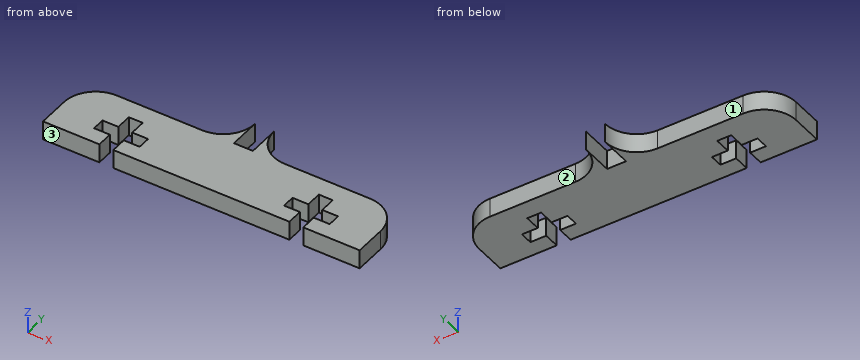
```python
from build123d import *

# Parameters (mm, degrees)
BOSS_EXTRUDE1_DEPTH = 3
FILLET1_R           = 5


with BuildPart() as part:
    # Sketch1 → Boss-Extrude1 (new body)
    with BuildSketch(Plane.XY):
        with BuildLine():
            Line((-25, -5), (-16.1, -5))
            Line((-16.1, -5), (-16.1, -2.5))
            Line((-16.1, -2.5), (-18.6, -2.5))
            Line((-18.6, -2.5), (-18.6, -0.5))
            Line((-18.6, -0.5), (-16.1, -0.5))
            Line((-16.1, -0.5), (-16.1, 2))
            Line((-16.1, 2), (-13.9, 2))
            Line((-13.9, 2), (-13.9, -0.5))
            Line((-13.9, -0.5), (-11.4, -0.5))
            Line((-11.4, -0.5), (-11.4, -2.5))
            Line((-11.4, -2.5), (-13.9, -2.5))
            Line((-13.9, -2.5), (-13.9, -5))
            Line((-13.9, -5), (13.9, -5))
            Line((13.9, -5), (13.9, -2.5))
            Line((13.9, -2.5), (11.4, -2.5))
            Line((11.4, -2.5), (11.4, -0.5))
            Line((11.4, -0.5), (13.9, -0.5))
            Line((13.9, -0.5), (13.9, 2))
            Line((13.9, 2), (16.1, 2))
            Line((16.1, 2), (16.1, -0.5))
            Line((16.1, -0.5), (18.6, -0.5))
            Line((18.6, -0.5), (18.6, -2.5))
            Line((18.6, -2.5), (16.1, -2.5))
            Line((16.1, -2.5), (16.1, -5))
            Line((16.1, -5), (25, -5))
            Line((25, -5), (25, 5))
            Line((25, 5), (6.5, 5))
            ThreePointArc((6.5, 5), (2.964466094, 6.464466094), (1.5, 10))
            Line((1.5, 10), (1.5, 5))
            Line((1.5, 5), (-1.5, 5))
            Line((-1.5, 5), (-1.5, 10))
            ThreePointArc((-1.5, 10), (-2.964466094, 6.464466094), (-6.5, 5))
            Line((-6.5, 5), (-25, 5))
            Line((-25, 5), (-25, -5))
        make_face()
    extrude(amount=BOSS_EXTRUDE1_DEPTH)

    # Fillet1
    fillet1_edges = [part.edges().sort_by_distance(p)[0] for p in [
        (25, 5, 1.5),
        (-25, 5, 1.5),
    ]]
    fillet(fillet1_edges, radius=FILLET1_R)


solid = part.part
```
For this review, take the finished solid that the model builds, in its own axes (mm). Face numbers are marked on the shaded views. A direction names the side the tool comes from. Give positions to 0.01 mm unless a question says otherwise; leave off trailing zeros. Write each loop counter-clockwise with the first axis right and the second up, starting at its lowest first coordinate (ties: lowest second). Pieces come first, ordered by that corner, then holes. Notation, with made-up numbers: M 59.25,17 L 82.25,17 A24 ccw 82.25,40 Z; hole C -4.5,-38 d5. An arc over 180 degrees is marked long. Answer as CSV lines item,"result".
1. Consider section D-D, the plane y = -4. Write out the cut boundary in (x, z), then the cut area to 3 significant figures.
Findings:
outline,"M -25,0 L -16.1,0 L -16.1,3 L -25,3 Z; M -13.9,0 L 13.9,0 L 13.9,3 L -13.9,3 Z; M 16.1,0 L 25,0 L 25,3 L 16.1,3 Z"
area,"137 mm2"
2. Wall thickness on line 1 (X direction, y = -3.75, z = 0.55); line 2 (X direction, y = 1.25, z = 0.7); line 3 (Y direction, x = -6.5, z = 1.65): over which ranges is each line inside the solid? List them lowest first.
Findings:
line 1,"x = -25 to -16.1, -13.9 to 13.9, 16.1 to 25"
line 2,"x = -24.84 to -16.1, -13.9 to 13.9, 16.1 to 24.84"
line 3,"y = -5 to 5"
3. Consider section C-C, the plane y = 8. Write out the cut boundary in (x, z), then the cut area to 3 significant figures.
Findings:
outline,"M -1.92,0 L -1.5,0 L -1.5,3 L -1.92,3 Z; M 1.5,0 L 1.92,0 L 1.92,3 L 1.5,3 Z"
area,"2.50 mm2"
4. For pin 1 (5 mm diameter, centred on x = 5.5, y = -0.5, fed in from -Z); pin 2 (0.7 mm diameter, centred on x = 15.5, z = 1.5, fed in from -Y); pin 3 (1.2 mm diameter, centred on x = -13, z = 1, fed in from +Y); pin 4 (1.5 mm diameter, centred on y = 3, z = 2.5, fed in from +X), all flat-tipped, find the tip position at first contact; note any pin that passes through.
Findings:
pin 1,"stops at z = 0"
pin 2,"stops at y = 2"
pin 3,"stops at y = 5"
pin 4,"stops at x = 24.47"
5. For the marked faces 1, 2 and 3, list the 3-axis set-ups (+Z, -Z, +X, -X, +Y, -Y) from which the entire face can be reached by the end or side of a thin tool; tool diameter is ignored.
Findings:
face 1,"+Z, -Z, -X, +Y"
face 2,"+Z, -Z, +X, +Y"
face 3,"+Z, -Z, +X, -X, -Y"
6. Consider section A-A, the plane x = -17.5. Write out the cut boundary in (y, z), then the cut area to 3 significant figures.
Findings:
outline,"M -5,0 L -2.5,0 L -2.5,3 L -5,3 Z; M -0.5,0 L 5,0 L 5,3 L -0.5,3 Z"
area,"24.0 mm2"
7. Consider section B-B, the plane y = -1.5. Write out the cut boundary in (x, z).
Findings:
outline,"M -25,0 L -18.6,0 L -18.6,3 L -25,3 Z; M -11.4,0 L 11.4,0 L 11.4,3 L -11.4,3 Z; M 18.6,0 L 25,0 L 25,3 L 18.6,3 Z"
